Geometry check sheet. Reference: the model listing, model coordinates, mm. A direction names the side the tool comes from. Round coordinates to 2 decimals unless told otherwise and drop trailing zeros. Loops run counter-clockwise (first coordinate to the right, second up) from the corner with the lowest first, then second, coordinate; pieces in that order, holes last. Notation, with made-up numbers: M 38,56 L 86,56 A25 ccw 86,81 Z; hole C -21.5,69 d7. An arc over 180 degrees is marked long. Use one line per item in the form item = value. Start each with the question number.
1. Set-up check for faces 4 (the flat face through (20, 19, -1)), 5 (the cylindrical face through (18.08, 2.6, 27.44)), 6 (the cylindrical face through (16.421, 9.86, 52.665)): record each of +Z, -Z, +X, -X, +Y, -Y from which the full face is reachable in a straight line by a thin tool's end or side.
2. Cross-section at D-D (z = 54). Record the boundary of the cut face in (x, y).
3. Go/stop test with flat-tipped pins: pin 1 (5 mm diameter, centred on x = 0.56, z = 20, fed in from +Y); pin 2 (2 mm diameter, centred on x = 20, y = 22, fed in from +Z); pin 3 (12 mm diameter, centred on x = 1.5, y = 13, fed in from -Z). Record where each tip stops, or that it passes through.
4. Material ranges on line 1 (X direction, y = 8, z = 54); line 2 (X direction, y = 24, z = -33); line 3 (X direction, y = 0.2, z = 20), recorded low to high.
5. Cross-section at B-B (y = 6.5). State how many separate pieces and enclosed holes the cut face has, then the cut area to 4 significant figures.
6. Cross-section at C-C (x = -10.5). Record the boundary of the cut face in (y, z).
7. Draft check along Z on faces 1 (the flat face through (-20, 19, -13)), 2 (the flat face through (0, 19, 47.65)), 3 (the cylindrical face through (-18.05, 2.57, 27.56)). Enter one of: pulls with the +Z half, pulls with the -Z half, needs draft (parallel to the pull), parting line crosses it, or undercut.
8. Cross-section at A-A (z = -20). Record the boundary of the cut face in (x, y) (3 decimals), then the cut area to 3 significant figures.
```python
from build123d import *

# Parameters (mm, degrees)
SKETCH1_W                                      = 42
SKETCH1_H                                      = 100
BOSS_EXTRUDE1_DEPTH                            = 2
BOSS_EXTRUDE2_DEPTH                            = 34
FILLET1_R                                      = 2
CUT_EXTRUDE1_REACH                             = 67.092
SKETCH3_W                                      = 42
SKETCH3_H                                      = 3
LPATTERN1_COUNT                                = 7
LPATTERN1_PITCH                                = 12
CSK_FOR_M3_FLAT_HEAD_MACHINE_SCREW1_AT_2_COUNT = 2
CSK_FOR_M3_FLAT_HEAD_MACHINE_SCREW1_AT_2_PITCH = 40
SKETCH7_W                                      = 42
SKETCH7_H                                      = 8
SKETCH7_R                                      = 1.4
BOSS_EXTRUDE3_DEPTH                            = 20
FILLET2_R                                      = 1


with BuildPart() as part:
    # Sketch1 → Boss-Extrude1 (new body)
    with BuildSketch(Plane(origin=(0, 0, 0), x_dir=(1, 0, 0), z_dir=(0, 1, 0))):
        Rectangle(SKETCH1_W, SKETCH1_H)
    extrude(amount=BOSS_EXTRUDE1_DEPTH)

    # Sketch2 → Boss-Extrude2 (add)
    with BuildSketch(Plane(origin=(0, 2, 0), x_dir=(1, 0, 0), z_dir=(0, 1, 0))):
        Polygon((-21, 50), (-18.65, 50), (-18.65, -47.65), (18.65, -47.65), (18.65, 50), (21, 50), (21, -50), (-21, -50), align=None)
    extrude(amount=BOSS_EXTRUDE2_DEPTH)

    # Fillet1
    fillet1_edges = [part.edges().sort_by_distance(p)[0] for p in [
        (18.65, 2, -1.175),
        (0, 2, 47.65),
        (18.65, 19, 47.65),
        (-18.65, 2, -1.175),
        (-18.65, 19, 47.65),
    ]]
    fillet(fillet1_edges, radius=FILLET1_R)

    # Cut-Extrude1: up to this face of the body (flat: up to its plane)
    cut_extrude1_end = Plane(part.part.faces().sort_by_distance((0, 2, -2.175))[0])
    # Sketch3 → Cut-Extrude1 (cut, up to the picked face)
    with BuildSketch(Plane(origin=(0, 36, 0), x_dir=(1, 0, 0), z_dir=(0, 1, 0)), mode=Mode.PRIVATE) as cut_extrude1_sk1:
        with Locations((0, 38.5)):
            Rectangle(SKETCH3_W, SKETCH3_H)
    cut_extrude1_tool1 = split(extrude(cut_extrude1_sk1.sketch, amount=-CUT_EXTRUDE1_REACH, mode=Mode.PRIVATE), bisect_by=cut_extrude1_end, keep=Keep.BOTH, mode=Mode.PRIVATE)
    cut_extrude1 = cut_extrude1_tool1.solids().sort_by(Axis((0, 36, -38.5), (0, -1, 0)))[0]
    add(cut_extrude1, mode=Mode.SUBTRACT)

    # LPattern1: Cut-Extrude1 ×7
    with Locations(*[(0, 0, i * LPATTERN1_PITCH) for i in range(1, LPATTERN1_COUNT)]):
        add(cut_extrude1, mode=Mode.SUBTRACT)

    # Sketch5 → CSK for M3 Flat Head Machine Screw1 (revolve, cut)
    with BuildSketch(Plane(origin=(0.560724051, 2, -20), x_dir=(0, 0, 1), z_dir=(1, 0, 0))):
        Polygon((0, 0), (0, 2), (1.6, 2), (1.6, 1.775), (3.375, 0), align=None)
    csk_for_m3_flat_head_machine_screw1 = revolve(axis=Axis((0.560724051, 8.35, -20), (0, -1, 0)), mode=Mode.SUBTRACT)

    # CSK for M3 Flat Head Machine Screw1 at 2: CSK for M3 Flat Head Machine Screw1 ×2
    with Locations(*[(0, 0, i * CSK_FOR_M3_FLAT_HEAD_MACHINE_SCREW1_AT_2_PITCH) for i in range(1, CSK_FOR_M3_FLAT_HEAD_MACHINE_SCREW1_AT_2_COUNT)]):
        add(csk_for_m3_flat_head_machine_screw1, mode=Mode.SUBTRACT)

    # Sketch7 → Boss-Extrude3 (add)
    with BuildSketch(Plane.XZ):
        with Locations((0, 54)):
            Rectangle(SKETCH7_W, SKETCH7_H)
        with Locations(Location((-16, 54, 0), (0, 0, 270))):
            Circle(SKETCH7_R, mode=Mode.SUBTRACT)
        with Locations(Location((16, 54, 0), (0, 0, 270))):
            Circle(SKETCH7_R, mode=Mode.SUBTRACT)
    extrude(amount=-BOSS_EXTRUDE3_DEPTH)

    # Fillet2
    fillet2_edges = [part.edges().sort_by_distance(p)[0] for p in [
        (18.65, 36, -20.5),
        (18.65, 36, -8.5),
        (18.65, 36, 3.5),
        (18.65, 36, 15.5),
        (18.65, 36, 27.5),
        (18.65, 36, 40.325),
        (-18.65, 36, 27.5),
        (-18.65, 36, 15.5),
        (-18.65, 36, 3.5),
        (-18.65, 36, -8.5),
        (-18.65, 36, -20.5),
        (-18.65, 36, -32.5),
        (18.65, 20, -50),
        (-18.65, 20, -50),
        (0, 36, 50),
        (18.65, 36, -45),
        (-21, 20, 54),
        (0, 20, 58),
        (-21, 10, 58),
        (21, 20, 54),
        (21, 10, 58),
        (0, 36, 47.65),
        (-18.65, 36, 40.325),
        (0, 2, -50),
        (18.064213562, 36, 47.064213562),
        (-18.064213562, 36, 47.064213562),
        (18.064213562, 2.585786438, -50),
        (-18.064213562, 2.585786438, -50),
        (18.65, 36, -32.5),
        (-18.65, 36, -45),
        (21, 28, 50),
        (-21, 28, 50),
    ]]
    fillet(fillet2_edges, radius=FILLET2_R)


solid = part.part
```
Reported:
q1.face_4 = +X, -X, +Y
q1.face_5 = -Z, +Y
q1.face_6 = +Y, -Y
q2.outline = M -21,0 L -17.4,0 L -17.4,20 L -20,20 A1 ccw -21,19 Z; M -14.6,0 L 14.6,0 L 14.6,20 L -14.6,20 Z; M 17.4,0 L 21,0 L 21,19 A1 ccw 20,20 L 17.4,20 Z
q3.pin_1 = 1.13
q3.pin_2 = 50
q3.pin_3 = 47.65
q4.line_1 = -21 to -17.4, -14.6 to 14.6, 17.4 to 21
q4.line_2 = -21 to -18.65, 18.65 to 21
q4.line_3 = -21 to -1.04, 2.16 to 21
q5.separate_pieces = 15
q5.enclosed_holes = 2
q5.area = 783.5 mm²
q6.outline = M 0,-50 L 1,-50 A1 ccw 2,-49 L 2,45.65 A2 cw 4,47.65 L 35,47.65 A1 ccw 36,48.65 L 36,49 A1 ccw 35,50 L 20,50 L 20,57 A1 ccw 19,58 L 0,58 Z
q7.face_1 = undercut
q7.face_2 = pulls with the -Z half
q7.face_3 = needs draft
q8.outline = M -21,0 L -1.039,0 L -1.039,0.225 L -2.814,2 L -16.65,2 A2 cw -18.65,4 L -18.65,35 A1 ccw -19.65,36 L -21,36 Z; M 2.161,0 L 21,0 L 21,36 L 19.65,36 A1 ccw 18.65,35 L 18.65,4 A2 cw 16.65,2 L 3.936,2 L 2.161,0.225 Z
q8.area = 236 mm²
